```python
from build123d import *

# Parameters (mm, degrees)
SKETCH1_W                                       = 152.4
SKETCH1_H                                       = 177.8
BOSS_EXTRUDE1_DEPTH                             = 12.7
CUT_EXTRUDE5_START                              = -1.9304
CUT_EXTRUDE5_OUTLINE_W                          = 127
CUT_EXTRUDE5_OUTLINE_H                          = 127
CUT_EXTRUDE5_DEPTH                              = 1.9304
SKETCH7_W                                       = 102.9208
SKETCH7_H                                       = 102.9208
BOSS_EXTRUDE2_DEPTH                             = 1.9304
SKETCH9_W                                       = 34.925
SKETCH9_H                                       = 19.05
CBORE_FOR_10_SOCKET_HEAD_CAP_SCREW1_D           = 5.1054
CBORE_FOR_10_SOCKET_HEAD_CAP_SCREW1_CBORE_D     = 9.525
CBORE_FOR_10_SOCKET_HEAD_CAP_SCREW1_CBORE_DEPTH = 4.826
CBORE_FOR_10_SOCKET_HEAD_CAP_SCREW2_D           = 5.1054
CBORE_FOR_10_SOCKET_HEAD_CAP_SCREW2_CBORE_D     = 9.525
CBORE_FOR_10_SOCKET_HEAD_CAP_SCREW2_CBORE_DEPTH = 4.826
F_4_40_TAPPED_HOLE1_D                           = 2.2606
F_4_40_TAPPED_HOLE1_DEPTH                       = 7.5946
F_4_40_TAPPED_HOLE1_TIP                         = 0.679152758
SKETCH25_R                                      = 3.302
CUT_EXTRUDE7_DEPTH                              = 3.175
MIRROR2_COPY_1_SKETCH_R                         = 3.302
MIRROR2_COPY_1_DEPTH                            = 3.175
SKETCH26_W                                      = 152.4
SKETCH26_H                                      = 12.7
CUT_EXTRUDE8_DEPTH                              = 1.27
SKETCH30_R                                      = 1.6129
CUT_EXTRUDE12_DEPTH                             = 33.02
SKETCH31_R                                      = 3.302
CUT_EXTRUDE13_DEPTH                             = 40.64
CUT_EXTRUDE15_DEPTH                             = 2.032
SKETCH37_R                                      = 34.925
CUT_EXTRUDE18_DEPTH                             = 118.580133678
CHAMFER2_SIZE                                   = 8.8646
SKETCH38_W                                      = 127
SKETCH38_H                                      = 127
SKETCH38_W_2                                    = 102.9208
SKETCH38_H_2                                    = 102.9208
BOSS_EXTRUDE3_DEPTH                             = 1.9304


# Read off the part's stored shape, not the designer's step: Cut-Extrude5
with BuildPart() as part:
    # Sketch1 → Boss-Extrude1 (new body)
    with BuildSketch(Plane.XY.offset(12.7)):
        Rectangle(SKETCH1_W, SKETCH1_H)
    extrude(amount=-BOSS_EXTRUDE1_DEPTH)

    # Cut-Extrude5 outline → Cut-Extrude5 (cut)
    with BuildSketch(Plane.XY.offset(12.7).offset(CUT_EXTRUDE5_START)):
        Rectangle(CUT_EXTRUDE5_OUTLINE_W, CUT_EXTRUDE5_OUTLINE_H)
    extrude(amount=CUT_EXTRUDE5_DEPTH, mode=Mode.SUBTRACT)

    # Sketch7 → Boss-Extrude2 (add)
    with BuildSketch(Plane.XY.offset(10.7696)):
        Rectangle(SKETCH7_W, SKETCH7_H)
    extrude(amount=BOSS_EXTRUDE2_DEPTH)

    # Sketch9 → Cut-Revolve1 (revolve, cut)
    with BuildSketch(Plane.XZ, mode=Mode.PRIVATE) as cut_revolve1_sk:
        with Locations((17.4625, 11.4808)):
            Rectangle(SKETCH9_W, SKETCH9_H)
    revolve(cut_revolve1_sk.sketch.rotate(Axis((0, 0, 21.0058), (0, 0, -1)), 180), axis=Axis((0, 0, 21.0058), (0, 0, -1)), mode=Mode.SUBTRACT)

    # Sketch10 → Cut-Revolve2 (revolve, cut)
    with BuildSketch(Plane(origin=(-16.51, 0, 0), x_dir=(0, 0, -1), z_dir=(1, 0, 0))):
        Polygon((-6.35, 76.2), (-8.3165188, 76.2), (-7.718188123, 70.325851431), (-7.026590967, 70.325851431), (-7.026590967, 63.019039257), (-8.89, 62.746717258), (-8.89, 29.272053652), (-6.35, 29.272053652), align=None)
    revolve(axis=Axis((-16.51, 29.272053652, 6.35), (0, 1, 0)), mode=Mode.SUBTRACT)

    # CBORE for #10 Socket Head Cap Screw1 (through all)
    with Locations(Plane(origin=(0, 0, 0), x_dir=(-1, 0, 0), z_dir=(0, 0, -1))):
        with Locations((0, 72.009), (0, -72.009)):
            CounterBoreHole(CBORE_FOR_10_SOCKET_HEAD_CAP_SCREW1_D / 2, CBORE_FOR_10_SOCKET_HEAD_CAP_SCREW1_CBORE_D / 2, CBORE_FOR_10_SOCKET_HEAD_CAP_SCREW1_CBORE_DEPTH)

    # CBORE for #10 Socket Head Cap Screw2 (through all)
    with Locations(Plane(origin=(0, 0, 0), x_dir=(-1, 0, 0), z_dir=(0, 0, -1))):
        with Locations((71.12, 0), (71.12, -72.009), (71.12, 72.009)):
            cbore_for_10_socket_head_cap_screw2 = CounterBoreHole(CBORE_FOR_10_SOCKET_HEAD_CAP_SCREW2_D / 2, CBORE_FOR_10_SOCKET_HEAD_CAP_SCREW2_CBORE_D / 2, CBORE_FOR_10_SOCKET_HEAD_CAP_SCREW2_CBORE_DEPTH)

    # #4-40 Tapped Hole1
    with Locations(Plane.XY.offset(12.7)):
        with Locations((-31.75, 31.75), (31.75, 31.75), (31.75, -31.75), (-31.75, -31.75)):
            Hole(F_4_40_TAPPED_HOLE1_D / 2, depth=F_4_40_TAPPED_HOLE1_DEPTH)
            with Locations((0, 0, -(F_4_40_TAPPED_HOLE1_DEPTH + F_4_40_TAPPED_HOLE1_TIP / 2))):  # 118° drill point
                Cone(0, F_4_40_TAPPED_HOLE1_D / 2, F_4_40_TAPPED_HOLE1_TIP, mode=Mode.SUBTRACT)

    # Sketch25 → Cut-Extrude7 (cut)
    with BuildSketch(Plane.XY.offset(12.7)):
        with Locations((-31.75, 31.75)):
            Circle(SKETCH25_R)
    cut_extrude7 = extrude(amount=-CUT_EXTRUDE7_DEPTH, mode=Mode.SUBTRACT)

    # Mirror1: Cut-Extrude7 across plane
    add(cut_extrude7.mirror(Plane(origin=(0, 0, 0), x_dir=(0, 0, 1), z_dir=(1, 0, 0))), mode=Mode.SUBTRACT)

    # Mirror2: Cut-Extrude7 across plane
    add(cut_extrude7.mirror(Plane.ZX), mode=Mode.SUBTRACT)

    # Mirror2 copy 1 sketch → Mirror2 copy 1 (cut)
    with BuildSketch(Plane(origin=(0, 0, 12.7), x_dir=(-1, 0, 0), z_dir=(0, 0, 1))):
        with Locations((-31.75, 31.75)):
            Circle(MIRROR2_COPY_1_SKETCH_R)
    extrude(amount=-MIRROR2_COPY_1_DEPTH, mode=Mode.SUBTRACT)

    # Sketch26 → Cut-Extrude8 (cut)
    with BuildSketch(Plane.XY.offset(12.7)):
        with Locations((0, 82.55)):
            Rectangle(SKETCH26_W, SKETCH26_H)
    cut_extrude8 = extrude(amount=-CUT_EXTRUDE8_DEPTH, mode=Mode.SUBTRACT)

    # Mirror4: Cut-Extrude8 across plane
    add(cut_extrude8.mirror(Plane.ZX), mode=Mode.SUBTRACT)

    # Sketch30 → Cut-Extrude12 (cut)
    with BuildSketch(Plane(origin=(0, 88.9, 0), x_dir=(1, 0, 0), z_dir=(0, 1, 0))):
        with Locations(Location((-7.762889406, -7.9375, 0), (0, 0, 270))):
            Circle(SKETCH30_R)
        with Locations(Location((-25.257110594, -7.9375, 0), (0, 0, 270))):
            Circle(SKETCH30_R)
    extrude(amount=-CUT_EXTRUDE12_DEPTH, mode=Mode.SUBTRACT)

    # Sketch31 → Cut-Extrude13 (cut)
    with BuildSketch(Plane(origin=(0, 88.9, 0), x_dir=(1, 0, 0), z_dir=(0, 1, 0))):
        with Locations(Location((-16.51, -6.35, 0), (0, 0, 270))):
            Circle(SKETCH31_R)
    extrude(amount=-CUT_EXTRUDE13_DEPTH, mode=Mode.SUBTRACT)

    # Mirror7: CBORE for #10 Socket Head Cap Screw2 across plane
    add(cbore_for_10_socket_head_cap_screw2.mirror(Plane(origin=(0, 0, 0), x_dir=(0, 0, 1), z_dir=(1, 0, 0))), mode=Mode.SUBTRACT)

    # Sketch33 → Cut-Extrude15 (cut)
    with BuildSketch(Plane(origin=(0, 0, 12.7), x_dir=(-1, 0, 0), z_dir=(0, 0, -1))):
        with BuildLine():
            Line((-62.7507, 67.6275), (62.7507, 67.6275))
            ThreePointArc((62.7507, 67.6275), (66.19911835, 66.19911835), (67.6275, 62.7507))
            Line((67.6275, 62.7507), (67.6275, -62.7507))
            ThreePointArc((67.6275, -62.7507), (66.19911835, -66.19911835), (62.7507, -67.6275))
            Line((62.7507, -67.6275), (-62.7507, -67.6275))
            ThreePointArc((-62.7507, -67.6275), (-66.19911835, -66.19911835), (-67.6275, -62.7507))
            Line((-67.6275, -62.7507), (-67.6275, 62.7507))
            ThreePointArc((-67.6275, 62.7507), (-66.19911835, 66.19911835), (-62.7507, 67.6275))
        make_face()
        with BuildLine():
            Line((-62.7507, 65.2907), (62.7507, 65.2907))
            ThreePointArc((62.7507, 65.2907), (64.546751224, 64.546751224), (65.2907, 62.7507))
            Line((65.2907, 62.7507), (65.2907, -62.7507))
            ThreePointArc((65.2907, -62.7507), (64.546751224, -64.546751224), (62.7507, -65.2907))
            Line((62.7507, -65.2907), (-62.7507, -65.2907))
            ThreePointArc((-62.7507, -65.2907), (-64.546751224, -64.546751224), (-65.2907, -62.7507))
            Line((-65.2907, -62.7507), (-65.2907, 62.7507))
            ThreePointArc((-65.2907, 62.7507), (-64.546751224, 64.546751224), (-62.7507, 65.2907))
        make_face(mode=Mode.SUBTRACT)
    extrude(amount=CUT_EXTRUDE15_DEPTH, mode=Mode.SUBTRACT)

    # Sketch37 → Cut-Extrude18 (cut, through all)
    with BuildSketch(Plane.XY.offset(1.9558)):
        with Locations(Location((0, 0, 0), (0, 0, 180))):
            Circle(SKETCH37_R)
    extrude(amount=-CUT_EXTRUDE18_DEPTH, mode=Mode.SUBTRACT)

    # Chamfer2
    # the kernel refuses this chamfer: 8.8646 mm, written as the material it takes off along each edge
    with BuildSketch(Plane(origin=(0, 0, 0), x_dir=(-1, 0, 0), z_dir=(0, 1, 0))) as chamfer2_piece_1:
        Polygon((34.925 + CHAMFER2_SIZE, 0), (34.925, CHAMFER2_SIZE), (34.925, 0), align=None)
    revolve(axis=Axis((0, 0, 0), (0, 0, 1)), mode=Mode.SUBTRACT)

    # Sketch38 → Boss-Extrude3 (add)
    with BuildSketch(Plane.XY.offset(10.7696)):
        Rectangle(SKETCH38_W, SKETCH38_H)
        Rectangle(SKETCH38_W_2, SKETCH38_H_2, mode=Mode.SUBTRACT)
    extrude(amount=BOSS_EXTRUDE3_DEPTH)


solid = part.part
```
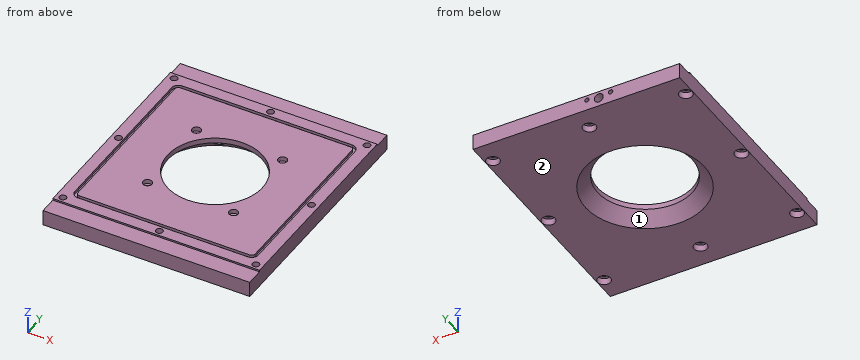
Check sheet for the modelled part. Datum: model origin and axes. Units: mm. Face numbers are marked on the shaded views. Give positions to 0.01 mm unless a question says otherwise; leave off trailing zeros. Loops run counter-clockwise (first coordinate to the right, second up) from the corner with the lowest first, then second, coordinate; pieces in that order, holes last. Notation, with made-up numbers: M 85,28.5 L 139,28.5 A21 cw 139,60.5 Z; hole C 83.5,12 d11. An arc over 180 degrees is marked long. Answer as CSV lines item,"result".
Item 1: Sectioned sample at B-B, the plane y = 59.5. Enter the section's corners in (x, z).
Reply:
outline,"M -76.2,0 L 76.2,0 L 76.2,12.7 L 67.63,12.7 L 67.63,10.67 L 65.29,10.67 L 65.29,12.7 L -65.29,12.7 L -65.29,10.67 L -67.63,10.67 L -67.63,12.7 L -76.2,12.7 Z; hole C -25.26,7.94 d3.23; hole C -16.51,6.35 d6.6; hole C -7.76,7.94 d3.23"
Item 2: Draft check along X on the marked faces 1 and 2. Enter one of: pulls with the +X half, pulls with the -X half, needs draft (parallel to the pull), parting line crosses it, or undercut.
Reply:
face 1,"undercut"
face 2,"needs draft"
Item 3: Depth check by flat-ended pin: pin 1 Ø1 at (x, z) = (31.5, 12) entering from -Y; pin 2 Ø1 at (x, z) = (-25.5, 8.5) entering from +Y. Enter the tip coordinate at first touch or a pass-through.
Reply:
pin 1,"y = -76.2"
pin 2,"y = 55.88"
Item 4: Scan lines: L1, parallel to Y at x = 60.5, z = 12; L2, parallel to Y at x = 9, z = 11; L3, parallel to X at y = -19.5, z = 12.25. Record each from-to range of solid material in increasing order.
Reply:
L1,"-76.2 to -67.63, -65.29 to 65.29, 67.63 to 76.2"
L2,"-88.9 to -67.63, -65.29 to -33.75, 33.75 to 65.29, 67.63 to 88.9"
L3,"-76.2 to -67.63, -65.29 to -28.97, 28.97 to 65.29, 67.63 to 76.2"
Item 5: Sectioned sample at C-C, the plane x = -59. Enter the section's corners in (y, z).
Reply:
outline,"M -88.9,0 L 88.9,0 L 88.9,11.43 L 76.2,11.43 L 76.2,12.7 L 67.63,12.7 L 67.63,10.67 L 65.29,10.67 L 65.29,12.7 L -65.29,12.7 L -65.29,10.67 L -67.63,10.67 L -67.63,12.7 L -76.2,12.7 L -76.2,11.43 L -88.9,11.43 Z"
Item 6: Sectioned sample at A-A, the plane x = 71.12. State how many separate pieces and enclosed holes the cut face has, then the cut area to 3 significant figures.
Reply:
separate pieces,"4"
enclosed holes,"0"
area,"1,970 mm^2"
